Geometry check sheet. Reference: the model listing, model coordinates, mm. A direction names the side the tool comes from. Coordinates: 2 decimals unless noted, no trailing zeros. Loops run counter-clockwise (first coordinate to the right, second up) from the corner with the lowest first, then second, coordinate; pieces in that order, holes last. Notation, with made-up numbers: (15.5, 38.25) - (65.5, 38.25) arc R31 ccw to (65.5, 77.25) - close; hole circle Ø7 at (-6.75, 76.5). An arc over 180 degrees is marked (long way). Write item = value, one per line. Start each with the question number.
from build123d import *

# Parameters (mm, degrees)
F1_DEPTH = 25.4


with BuildPart() as f1:
    # F0 (on Top) → F1 (new body)
    with BuildSketch(Plane.XY):
        with BuildLine():
            ThreePointArc((-47.917716, 13.608789), (-45.857251, 7.887993), (-40.276696, 5.473362))
            Line((-40.276696, 5.473362), (-1.308659, 5.473362))
            ThreePointArc((-1.308659, 5.473362), (0.14184, 6.648248), (-1.131254, 8.013362))
            Line((-1.131254, 8.013362), (-30.934975, 8.013362))
            ThreePointArc((-30.934975, 8.013362), (-32.686526, 8.926962), (-32.939632, 10.886179))
            Line((-32.939632, 10.886179), (-12.666556, 66.03077))
            ThreePointArc((-12.666556, 66.03077), (-14.397306, 75.64713), (-23.704619, 78.620983))
            ThreePointArc((-23.704619, 78.620983), (-24.659504, 77.139495), (-23.216566, 76.127298))
            ThreePointArc((-23.216566, 76.127298), (-16.365183, 74.040443), (-15.011284, 67.007424))
            Line((-15.011284, 67.007424), (-35.468568, 11.361769))
            ThreePointArc((-35.468568, 11.361769), (-41.409662, 8.133505), (-45.376973, 13.608789))
            ThreePointArc((-45.376973, 13.608789), (-46.647345, 15.004164), (-47.917716, 13.608789))
        make_face()
    extrude(amount=F1_DEPTH)


solid = f1.part
(1) Depth check by flat-ended pin: pin 1 (1 mm diameter, centred on y = 66, z = 21, fed in from -X); pin 2 (8 mm diameter, centred on x = -29.5, z = 5, fed in from -Y); pin 3 (12.5 mm diameter, centred on x = -11, z = 18, fed in from +Y). Enter the tip coordinate at first touch or a pass-through.
(2) Sectioned sample at A-A on x = -21. Enter the section's corners in (y, z), plus the area to 3 significant figures.
(3) Sectioned sample at B-B on x = -27. Enter the section's corners in (y, z).
(4) Tool access check on faces 1 (the face through (-26, 31, 25.4)), 2 (the face through (-16, 8.013, 13)). Record the directions out of +Z, -Z, +X, -X, +Y, -Y that give a thin tool (end or side, any length) a straight path to the whole face; none if there is none.
(5) Sectioned sample at D-D on y = 21. Enter the section's corners in (x, z), plus the area to 3 significant figures.
(6) Scan lines: line 1 (Y direction, x = -10.5, z = 16.75); line 2 (Y direction, x = -39, z = 10.75); line 3 (X direction, y = 56.5, z = 9). Record each from-to range of solid material in increasing order.
(7) Draft check along Y on faces 3 (the face through (-14.303, 75.538, 12.522)), 4 (the face through (-16.44, 74.12, 12.52)), 5 (the face through (-21, 5.473, 13)), 6 (the face through (-26, 31, 0)). Enter one of: pulls with the +Y half, pulls with the -Y half, needs draft (parallel to the pull), parting line crosses it, or undercut.
(8) Sectioned sample at C-C on z = 9.75. Enter the section's corners in (x, y), plus the area to 3 significant figures.
Working result:
q1.pin_1 = -15.57
q1.pin_2 = 5.47
q1.pin_3 = 77.86
q2.outline = (5.47, 0) - (8.01, 0) - (8.01, 25.4) - (5.47, 25.4) - close; (43.36, 0) - (50.72, 0) - (50.72, 25.4) - (43.36, 25.4) - close; (76.32, 0) - (78.86, 0) - (78.86, 25.4) - (76.32, 25.4) - close
q2.area = 316 mm2
q3.outline = (5.47, 0) - (8.01, 0) - (8.01, 25.4) - (5.47, 25.4) - close; (27.04, 0) - (34.4, 0) - (34.4, 25.4) - (27.04, 25.4) - close
q4.face_1 = +Z, +X, -X, +Y, -Y
q4.face_2 = +Z, -Z, +X
q5.outline = (-31.93, 0) - (-29.22, 0) - (-29.22, 25.4) - (-31.93, 25.4) - close
q5.area = 68.7 mm2
q6.line_1 = 5.47 to 8.01
q6.line_2 = 5.47 to 8.17
q6.line_3 = -18.87 to -16.17
q7.face_3 = undercut
q7.face_4 = undercut
q7.face_5 = pulls with the -Y half
q7.face_6 = needs draft
q8.outline = (-47.92, 13.61) arc R7.66 ccw to (-40.28, 5.47) - (-1.31, 5.47) arc R1.28 ccw (long way) to (-1.13, 8.01) - (-30.93, 8.01) arc R2.14 cw to (-32.94, 10.89) - (-12.67, 66.03) arc R9.47 ccw to (-23.7, 78.62) arc R1.27 ccw to (-23.22, 76.13) arc R6.94 cw to (-15.01, 67.01) - (-35.47, 11.36) arc R5.12 cw to (-45.38, 13.61) arc R1.28 ccw (long way) to start
q8.area = 342 mm2
